Geometry: see drawing. Coordinates: mm, zero at the bounding-box minimum. A direction names the side the tool comes from. Coordinates: 2 decimals unless noted, no trailing zeros. Write each loop counter-clockwise with the first axis right and the second up, starting at its lowest first coordinate (ties: lowest second). Pieces come first, ordered by that corner, then holes. Notation, with made-up numbers: M 13.25,76 L 17.25,76 A23 ccw 17.25,97 Z; hole C -26,55 d10. An arc over 180 degrees is marked long. Answer as CSV lines item,"result". Start each with the question number.
1. Reachability of the marked faces 1 and 2 from +Z, -Z, +X, -X, +Y, -Y: full face, straight path, thin tool, end or side. Return the list, or none.
2. Section A-A on x = 54. Return the cut outline in (y, z) (3 decimals).
3. Section C-C on z = 11.5. Return the cut outline in (x, y) (3 decimals), plus the area to 3 significant figures.
4. Mould query, pull axis X, two halves, no side actions, for the marked faces 3, 4 and 5. Classes: pulls with the +X half, pulls with the -X half, needs draft (parallel to the pull), parting line crosses it, or undercut.
5. Section B-B on y = 23.5. Return the cut outline in (x, z), plus the area to 3 significant figures.
6. Line query: probe 1 along Y at (x, z) = (49.5, 4.25) (3 decimals); probe 2 along Y at (x, z) = (68.5, 3.25) (3 decimals); probe 3 along Z at (x, y) = (34.5, 58). Output: solid intervals per line, ascending. Write a range as [from, to].
7. Contact query for flat-ended pins moving along their axis: pin 1 Ø1.5 at (y, z) = (71, 17.5) entering from -X; pin 2 Ø10 at (y, z) = (28.5, 4.5) entering from +X; pin 3 Ø10 at (x, z) = (36.5, 10.5) entering from +Y; pin 4 Ø22.5 at (x, y) = (26.5, 22) entering from -Z. Output: stop coordinate, or through.
8. Section D-D on x = 44. Return the cut outline in (y, z) (1 decimal), plus the area to 3 significant figures.
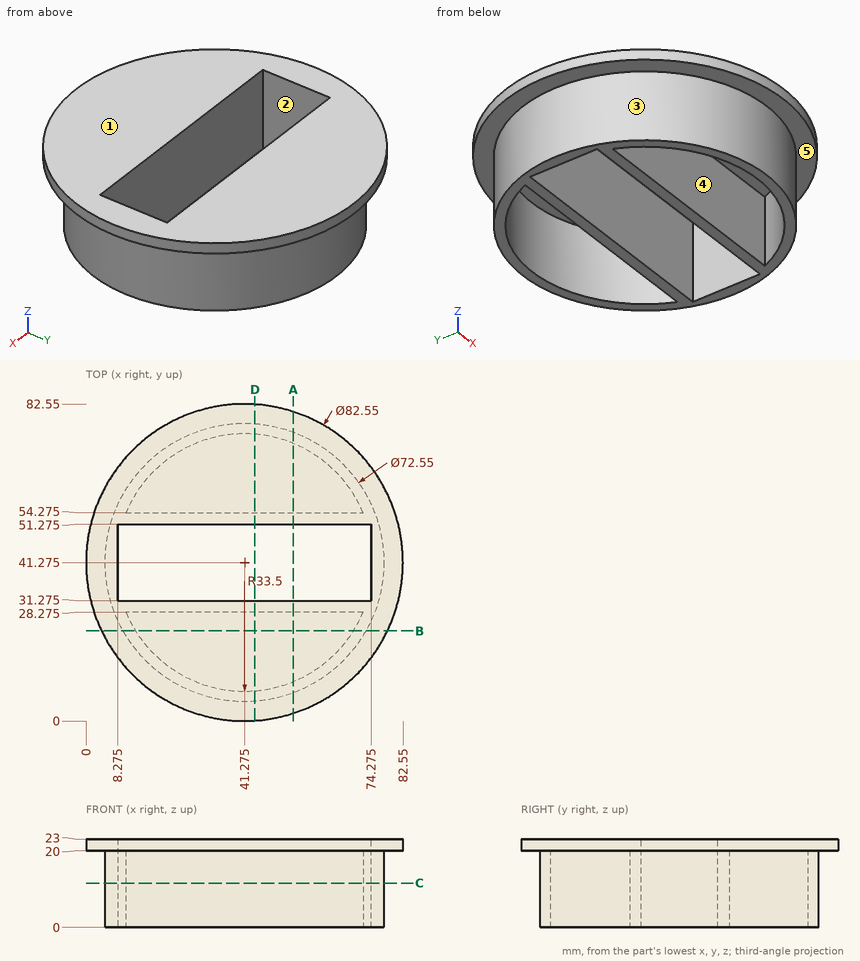
Values:
1,face 1,"+Z, +X, -X, +Y, -Y"
1,face 2,"+Z, -Z"
2,outline,"M 2.011,20 L 7.305,20 L 7.305,0 L 10.286,0 L 10.286,20 L 28.275,20 L 28.275,0 L 31.275,0 L 31.275,23 L 2.011,23 Z; M 51.275,0 L 54.275,0 L 54.275,20 L 72.264,20 L 72.264,0 L 75.245,0 L 75.245,20 L 80.539,20 L 80.539,23 L 51.275,23 Z"
3,outline,"C 41.275,41.275 d72.55; hole M 8.275,31.275 L 74.275,31.275 L 74.275,51.275 L 8.275,51.275 Z; hole M 10.4,28.275 A33.5 ccw 72.15,28.275 Z; hole M 10.4,54.275 L 72.15,54.275 A33.5 ccw Z"
3,area,"986 mm²"
4,face 3,"parting line crosses it"
4,face 4,"undercut"
4,face 5,"needs draft"
5,outline,"M 4.02,20 L 9.65,20 L 9.65,0 L 12.88,0 L 12.88,20 L 69.67,20 L 69.67,0 L 72.9,0 L 72.9,20 L 78.53,20 L 78.53,23 L 4.02,23 Z"
5,area,"353 mm²"
6,probe 1,"[5.945, 8.8], [28.275, 31.275], [51.275, 54.275], [73.75, 76.605]"
6,probe 2,"[17.303, 21.755], [28.275, 31.275], [51.275, 54.275], [60.795, 65.247]"
6,probe 3,"[20, 23]"
7,pin 1,"x = 19.45"
7,pin 2,"x = 76.71"
7,pin 3,"y = 77.55"
7,pin 4,"z = 0"
8,outline,"M 0.1,20 L 5.1,20 L 5.1,0 L 7.9,0 L 7.9,20 L 28.3,20 L 28.3,0 L 31.3,0 L 31.3,23 L 0.1,23 Z; M 51.3,0 L 54.3,0 L 54.3,20 L 74.7,20 L 74.7,0 L 77.4,0 L 77.4,20 L 82.5,20 L 82.5,23 L 51.3,23 Z"
8,area,"418 mm²"
